from build123d import *

# Parameters (mm, degrees)
BOSS_EXTRUDE1_DEPTH = 4.75
BOSS_EXTRUDE2_DEPTH = 0.76
LPATTERN1_COUNT     = 3
LPATTERN1_PITCH     = 2.54
LPATTERN1_COL_COUNT = 2
LPATTERN1_COL_PITCH = 2.54


with BuildPart() as part:
    # Sketch1 → Boss-Extrude1 (new, symmetric)
    with BuildSketch(Plane.XY):
        Polygon((3.076266246, 1.7), (-3.076266246, 1.7), (-3.285, 0), (-3.076266246, -1.7), (3.076266246, -1.7), (3.285, 0), align=None)
    extrude(amount=BOSS_EXTRUDE1_DEPTH, both=True)

    # Sketch2 → Boss-Extrude2 (add, symmetric)
    with BuildSketch(Plane.XY.offset(1.27)):
        with BuildLine():
            Line((0, 0), (3.924366416, 0))
            ThreePointArc((3.924366416, 0), (3.984689335, -0.02024321), (4.020589663, -0.07277709))
            Line((4.020589663, -0.07277709), (4.85, -3.004445821))
            ThreePointArc((4.85, -3.004445821), (4.921800656, -3.10951358), (5.042446493, -3.15))
            Line((5.042446493, -3.15), (5.35, -3.15))
            Line((5.35, -3.15), (5.35, -2.85))
            Line((5.35, -2.85), (5.118080076, -2.85))
            Line((5.118080076, -2.85), (4.309259402, 0.008891642))
            ThreePointArc((4.309259402, 0.008891642), (4.16565809, 0.219027159), (3.924366416, 0.3))
            Line((3.924366416, 0.3), (0, 0.3))
            Line((0, 0.3), (-3.924366416, 0.3))
            ThreePointArc((-3.924366416, 0.3), (-4.16565809, 0.219027159), (-4.309259402, 0.008891642))
            Line((-4.309259402, 0.008891642), (-5.118080076, -2.85))
            Line((-5.118080076, -2.85), (-5.35, -2.85))
            Line((-5.35, -2.85), (-5.35, -3.15))
            Line((-5.35, -3.15), (-5.042446493, -3.15))
            ThreePointArc((-5.042446493, -3.15), (-4.921800656, -3.10951358), (-4.85, -3.004445821))
            Line((-4.85, -3.004445821), (-4.020589663, -0.07277709))
            ThreePointArc((-4.020589663, -0.07277709), (-3.984689335, -0.02024321), (-3.924366416, 0))
            Line((-3.924366416, 0), (0, 0))
        make_face()
    boss_extrude2 = extrude(amount=BOSS_EXTRUDE2_DEPTH, both=True)

    # LPattern1: Boss-Extrude2 ×3
    with Locations(*[(0, 0, -i * LPATTERN1_PITCH) for i in range(1, LPATTERN1_COUNT)]):
        add(boss_extrude2)

    # LPattern1 col: Boss-Extrude2 ×2
    with Locations(*[(0, 0, i * LPATTERN1_COL_PITCH) for i in range(1, LPATTERN1_COL_COUNT)]):
        add(boss_extrude2)


solid = part.part
Verification items for the finished model (mm, model axes). Give positions to 0.01 mm unless a question says otherwise; leave off trailing zeros. Write each loop counter-clockwise with the first axis right and the second up, starting at its lowest first coordinate (ties: lowest second). Pieces come first, ordered by that corner, then holes. Notation, with made-up numbers: M 45.5,18 L 54.5,18 A23 cw 54.5,48 Z; hole C -21,26 d6. An arc over 180 degrees is marked long. Put each result on its own line as item: value. Start each with the question number.
1. Section check B-B (y = -1.85). Give the number of separate pieces and of enclosed holes in the cut face, and give its area (3 significant figures).
2. Section check C-C (z = 2.5). Record the cut outline in (x, y) (3 decimals), and give its area (3 significant figures).
3. Section check A-A (x = 3.75). Record the cut outline in (y, z).
4. Go/stop test with flat-tipped pins: pin 1 Ø1 at (y, z) = (0.5, -1.5) entering from +X; pin 2 Ø1.1 at (x, y) = (-5, -1) entering from -Z; pin 3 Ø2.5 at (x, y) = (4.5, -2) entering from +Z. Record where each tip stops, or that it passes through.
5. Draft check along X on faces 1 (the face through (-3.18, -0.84, 0.07)), 2 (the face through (-4.708, -1.401, -1.259)), 3 (the face through (4.72, -1.44, 3.82)), 4 (the face through (4.43, -1.52, -1.26)). Enter one of: +X half, -X half, draft (parallel to the pull), parting line (faces both ways), or undercut.
6. Scan lines: line 1 along Y through (x, z) = (-0.25, -3); line 2 along X through (y, z) = (-2.15, -4); line 3 along X through (y, z) = (-2.3, -3.25). Record each from-to range of solid material in increasing order. Write a range as [from, to].
7. Section check D-D (x = -2). Record the cut outline in (y, z).
Answer list:
1. separate pieces: 8
1. enclosed holes: 0
1. area: 3.79 mm2
2. outline: M -3.285,0 L -3.076,-1.7 L 3.076,-1.7 L 3.285,0 L 3.076,1.7 L -3.076,1.7 Z
2. area: 21.6 mm2
3. outline: M 0,-4.57 L 0.3,-4.57 L 0.3,-3.05 L 0,-3.05 Z; M 0,-2.03 L 0.3,-2.03 L 0.3,-0.51 L 0,-0.51 Z; M 0,0.51 L 0.3,0.51 L 0.3,2.03 L 0,2.03 Z; M 0,3.05 L 0.3,3.05 L 0.3,4.57 L 0,4.57 Z
4. pin 1: x = 4.31
4. pin 2: z = -4.57
4. pin 3: z = 4.57
5. face 1: undercut
5. face 2: -X half
5. face 3: +X half
5. face 4: undercut
6. line 1: [-1.7, 1.7]
6. line 2: [-4.92, -4.61], [4.61, 4.92]
6. line 3: [-4.96, -4.65], [4.65, 4.96]
7. outline: M -1.7,-4.75 L 1.7,-4.75 L 1.7,4.75 L -1.7,4.75 Z
